from build123d import *

# Parameters (mm, degrees)
SKETCH_1_W          = 19
SKETCH_1_H          = 20
EXTRUDE_1_DEPTH     = 5
SKETCH_2_R          = 1.65
CUT_EXTRUDE_1_DEPTH = 15.671400751
FILLET_1_R          = 2
SKETCH_3_R          = 5
CUT_EXTRUDE_2_DEPTH = 10


with BuildPart() as part:
    # 草图1 → 凸台-拉伸1 (new body)
    with BuildSketch(Plane(origin=(0, 0, 0), x_dir=(1, 0, 0), z_dir=(0, 1, 0))):
        Rectangle(SKETCH_1_W, SKETCH_1_H)
    extrude(amount=EXTRUDE_1_DEPTH)

    # 草图2 → 切除-拉伸1 (cut, through all)
    with BuildSketch(Plane(origin=(0, 5, 0), x_dir=(1, 0, 0), z_dir=(0, 1, 0))):
        with Locations(Location((-5, 7.5, 0), (0, 0, 270))):
            Circle(SKETCH_2_R)
        with Locations(Location((5, 7.5, 0), (0, 0, 270))):
            Circle(SKETCH_2_R)
        with Locations(Location((5, -7.5, 0), (0, 0, 90))):
            Circle(SKETCH_2_R)
        with Locations(Location((-5, -7.5, 0), (0, 0, 90))):
            Circle(SKETCH_2_R)
    extrude(amount=-CUT_EXTRUDE_1_DEPTH, mode=Mode.SUBTRACT)

    # 圆角1
    fillet_1_edges = [part.edges().sort_by_distance(p)[0] for p in [
        (9.5, 2.5, 10),
        (-9.5, 2.5, 10),
        (-9.5, 2.5, -10),
        (9.5, 2.5, -10),
    ]]
    fillet(fillet_1_edges, radius=FILLET_1_R)

    # 草图3 → 切除-拉伸2 (cut)
    with BuildSketch(Plane(origin=(0, 5, 0), x_dir=(1, 0, 0), z_dir=(0, 1, 0))):
        with Locations(Location((0, 0, 0), (0, 0, 270))):
            Circle(SKETCH_3_R)
    extrude(amount=-CUT_EXTRUDE_2_DEPTH, mode=Mode.SUBTRACT)


solid = part.part
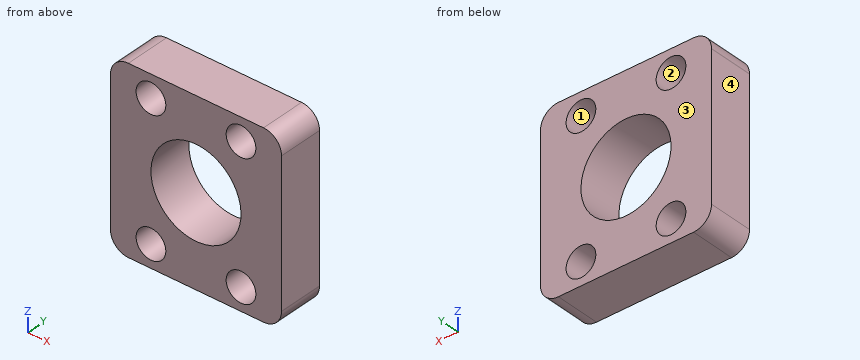
For this review, take the finished solid that the model builds, in its own axes (mm). Face numbers are marked on the shaded views. Round coordinates to 2 decimals unless told otherwise and drop trailing zeros. Loops run counter-clockwise (first coordinate to the right, second up) from the corner with the lowest first, then second, coordinate; pieces in that order, holes last. Notation, with made-up numbers: (-39, 12.25) - (15, 12.25) arc R23 ccw to (15, 27.25) - close; hole circle Ø8 at (-34, -3.5). An arc over 180 degrees is marked (long way). One line per question, with ' | ' between items.
Q1. The part is to be moulded in two halves that separate along X. For the marked faces 1, 2, 3 and 4, say which applies: released by +X, released by -X, zero draft, split by the parting line, or undercut.
Taken from the geometry:
face 1: undercut | face 2: undercut | face 3: zero draft | face 4: released by -X
Q2. Take a section at D-D (y = 1.1). Give the boundary of the cut face in (x, z).
Taken from the geometry:
outline: (-9.5, -8) arc R2 ccw to (-7.5, -10) - (7.5, -10) arc R2 ccw to (9.5, -8) - (9.5, 8) arc R2 ccw to (7.5, 10) - (-7.5, 10) arc R2 ccw to (-9.5, 8) - close; hole circle Ø3.3 at (-5, -7.5); hole circle Ø3.3 at (-5, 7.5); hole circle Ø10 at (0, 0); hole circle Ø3.3 at (5, -7.5); hole circle Ø3.3 at (5, 7.5)
Q3. Take a section at B-B (x = 0). Give the boundary of the cut face in (y, z), and give its area (3 significant figures).
Taken from the geometry:
outline: (0, -10) - (5, -10) - (5, -5) - (0, -5) - close; (0, 5) - (5, 5) - (5, 10) - (0, 10) - close | area: 50.0 mm²
Q4. Take a section at C-C (z = 7.5). Give the boundary of the cut face in (x, y).
Taken from the geometry:
outline: (-9.5, 0) - (-6.65, 0) - (-6.65, 5) - (-9.5, 5) - close; (-3.35, 0) - (3.35, 0) - (3.35, 5) - (-3.35, 5) - close; (6.65, 0) - (9.5, 0) - (9.5, 5) - (6.65, 5) - close
Q5. For pin 1 (2 mm diameter, centred on x = 5, z = 7.5, fed in from -Y), flat-tipped, find the tip position at first contact; note if it passes through.
Taken from the geometry:
pin 1: passes through
Q6. For line 1 along X through (y, z) = (2.7, 7.5); line 2 along X through (y, z) = (1.15, 0); line 3 along X through (y, z) = (0.7, 6.25), list the stretches that pass through material, from the lowest coordinate up. Write a range as [from, to].
Taken from the geometry:
line 1: x = [-9.5, -6.65], [-3.35, 3.35], [6.65, 9.5] | line 2: x = [-9.5, -5], [5, 9.5] | line 3: x = [-9.5, -6.08], [-3.92, 3.92], [6.08, 9.5]
Q7. Take a section at A-A (z = 0). Give the boundary of the cut face in (x, y).
Taken from the geometry:
outline: (-9.5, 0) - (-5, 0) - (-5, 5) - (-9.5, 5) - close; (5, 0) - (9.5, 0) - (9.5, 5) - (5, 5) - close
